Read the model definition and answer for the solid it produces. Units are mm, in the model's axes. A direction names the side the tool comes from. Round coordinates to 2 decimals unless told otherwise and drop trailing zeros. Loops run counter-clockwise (first coordinate to the right, second up) from the corner with the lowest first, then second, coordinate; pieces in that order, holes last. Notation, with made-up numbers: M 64.25,54.25 L 90.25,54.25 A23 ccw 90.25,65.25 Z; hole C 51,-5.75 d2. An arc over 180 degrees is marked long. Write each question's results on one line, items separated by ' | '.
from build123d import *

# Parameters (mm, degrees)
F0_W     = 48
F0_H     = 63
F0_R     = 2.25
F1_DEPTH = 2


with BuildPart() as f1:
    # F0 (on Front) → F1 (new body)
    with BuildSketch(Plane.XZ):
        with Locations((24, 31.5)):
            Rectangle(F0_W, F0_H)
        with Locations((4.319704, 4.899902)):
            Circle(F0_R, mode=Mode.SUBTRACT)
        with BuildLine():
            ThreePointArc((11.502249, 23.937898), (9.502249, 25.937898), (11.502249, 27.937898))
            Line((11.502249, 27.937898), (35.620832, 27.937898))
            ThreePointArc((35.620832, 27.937898), (37.620832, 25.937898), (35.620832, 23.937898))
            Line((35.620832, 23.937898), (11.502249, 23.937898))
        make_face(mode=Mode.SUBTRACT)
        with Locations((42.319704, 4.899902)):
            Circle(F0_R, mode=Mode.SUBTRACT)
        with BuildLine():
            ThreePointArc((11.620832, 29.937898), (8.620832, 32.937898), (11.620832, 35.937898))
            Line((11.620832, 35.937898), (35.620832, 35.937898))
            ThreePointArc((35.620832, 35.937898), (38.620832, 32.937898), (35.620832, 29.937898))
            Line((35.620832, 29.937898), (11.620832, 29.937898))
        make_face(mode=Mode.SUBTRACT)
        with BuildLine():
            ThreePointArc((12.296626, 37.937898), (10.296626, 39.937898), (12.296626, 41.937898))
            Line((12.296626, 41.937898), (35.302188, 41.937898))
            ThreePointArc((35.302188, 41.937898), (37.302188, 39.937898), (35.302188, 37.937898))
            Line((35.302188, 37.937898), (12.296626, 37.937898))
        make_face(mode=Mode.SUBTRACT)
        with Locations((5.310922, 57.899902)):
            Circle(F0_R, mode=Mode.SUBTRACT)
        with Locations((43.310922, 57.899902)):
            Circle(F0_R, mode=Mode.SUBTRACT)
    extrude(amount=F1_DEPTH)


solid = f1.part
Item 1: For faces 1 (the face through (23, -1, 35.938)), 2 (the face through (0, -1, 31)), determine the directions among +Z, -Z, +X, -X, +Y, -Y from which every point of the face is accessible in a straight line to the end or side of a thin tool.
Outcome:
face 1: +Y, -Y | face 2: +Z, -Z, -X, +Y, -Y
Item 2: The part is cut by section B-B (z = 39). Determine the outline of the cut face in (x, y).
Outcome:
outline: M 0,-2 L 10.53,-2 L 10.53,0 L 0,0 Z; M 37.07,-2 L 48,-2 L 48,0 L 37.07,0 Z
Item 3: Straight lines are drawn through the part: line 1 (Z direction, x = 34, y = -1.5); line 2 (Z direction, x = 3.5, y = -1.4); line 3 (X direction, y = -0.75, z = 5.5). For each, find the intervals that lie inside material, in ascending order.
Outcome:
line 1: z = 0 to 23.94, 27.94 to 29.94, 35.94 to 37.94, 41.94 to 63 | line 2: z = 0 to 2.8, 7 to 56.56, 59.24 to 63 | line 3: x = 0 to 2.15, 6.49 to 40.15, 44.49 to 48
Item 4: The part is cut by section C-C (y = -0.35). Determine the outline of the cut face in (x, z), plus the area to 3 significant figures.
Outcome:
outline: M 0,0 L 48,0 L 48,63 L 0,63 Z; hole C 4.32,4.9 d4.5; hole C 5.31,57.9 d4.5; hole M 11.5,23.94 L 35.62,23.94 A2 ccw 35.62,27.94 L 11.5,27.94 A2 ccw Z; hole M 11.62,29.94 L 35.62,29.94 A3 ccw 35.62,35.94 L 11.62,35.94 A3 ccw Z; hole M 12.3,37.94 L 35.3,37.94 A2 ccw 35.3,41.94 L 12.3,41.94 A2 ccw Z; hole C 42.32,4.9 d4.5; hole C 43.31,57.9 d4.5 | area: 2,570 mm2
Item 5: A flat-ended cylindrical pin translates along its axis: pin 1 (2.5 mm diameter, centred on x = 5.31, z = 57.9, fed in from -Y). Find the tip coordinate at first contact, or state that the pin passes through.
Outcome:
pin 1: passes through
Item 6: The part is cut by section A-A (x = 31). Determine the outline of the cut face in (y, z), plus the area to 3 significant figures.
Outcome:
outline: M -2,0 L 0,0 L 0,23.94 L -2,23.94 Z; M -2,27.94 L 0,27.94 L 0,29.94 L -2,29.94 Z; M -2,35.94 L 0,35.94 L 0,37.94 L -2,37.94 Z; M -2,41.94 L 0,41.94 L 0,63 L -2,63 Z | area: 98.0 mm2
